from build123d import *

# Parameters (mm, degrees)
F1_DEPTH = 254


with BuildPart() as f1:
    # F0 (on Top) → F1 (new body)
    with BuildSketch(Plane.XY):
        with BuildLine():
            ThreePointArc((-29.842062, 64.568127), (-16.660152, 69.246382), (-2.831554, 71.348459))
            Line((-2.831554, 71.348459), (63.255093, 33.106133))
            ThreePointArc((63.255093, 33.106133), (68.338603, 20.057423), (70.860705, 6.282449))
            Line((70.860705, 6.282449), (70.630319, 6.282449))
            Line((70.630319, 6.282449), (62.698711, 6.291514))
            Line((62.698711, 6.291514), (62.698711, 3.370512))
            Line((62.698711, 3.370512), (70.62698, 3.361451))
            Line((70.62698, 3.361451), (71.05381, 3.361451))
            Line((71.05381, 3.361451), (71.05343, 2.472453))
            Line((71.05343, 2.472453), (71.051259, -2.607547))
            Line((71.051259, -2.607547), (72.340575, -2.607547))
            Line((72.340575, -2.607547), (72.340575, 2.472453))
            Line((72.340575, 2.472453), (73.630904, 2.472453))
            ThreePointArc((73.630904, 2.472453), (70.963492, 20.100215), (64.273057, 36.625686))
            Line((64.273057, 36.625686), (-0.291446, 73.98688))
            ThreePointArc((-0.291446, 73.98688), (-20.379161, 70.861714), (-38.925678, 62.53647))
            Line((-38.925678, 62.53647), (-38.293981, 61.433763))
            Line((-38.293981, 61.433763), (-33.886026, 63.958903))
            Line((-33.886026, 63.958903), (-33.259961, 62.866025))
            ThreePointArc((-33.259961, 62.866025), (-32.867158, 63.073001), (-32.473114, 63.277605))
            Line((-32.473114, 63.277605), (-32.256725, 62.907915))
            Line((-32.256725, 62.907915), (-28.302588, 56.041036))
            Line((-28.302588, 56.041036), (-25.77126, 57.498644))
            Line((-25.77126, 57.498644), (-29.725397, 64.365523))
            Line((-29.725397, 64.365523), (-29.842062, 64.568127))
        make_face()
    extrude(amount=F1_DEPTH)


solid = f1.part
Read the model definition and answer for the solid it produces. Units are mm, in the model's axes. A direction names the side the tool comes from. Give positions to 0.01 mm unless a question says otherwise; leave off trailing zeros. Loops run counter-clockwise (first coordinate to the right, second up) from the corner with the lowest first, then second, coordinate; pieces in that order, holes last. Notation, with made-up numbers: M -35,9.25 L -2,9.25 A23 cw -2,24.25 Z; hole C -17,-19.75 d9. An arc over 180 degrees is marked long. Write each question's results on one line, items separated by ' | '.
1. The mould has two halves that part along X. Classify faces 1 (the face through (-20.11, 70.94, 125.22)), 2 (the face through (72.341, 0, 125)), 3 (the face through (30, 53, 254)), 4 (the face through (-36.12, 62.68, 125.22)): pulls with the +X half, pulls with the -X half, needs draft (parallel to the pull), parting line crosses it, or undercut.
Values:
face 1: pulls with the -X half | face 2: pulls with the +X half | face 3: needs draft | face 4: undercut
2. Straight lines are drawn through the part: line 1 (X direction, y = 0.5, z = 45); line 2 (X direction, y = 65, z = 206); line 3 (X direction, y = 66, z = 89). For each, find the intervals that lie inside material, in ascending order. Write a range as [from, to].
Values:
line 1: x = [71.05, 72.34] | line 2: x = [-34.66, -28.9], [8.14, 15.24] | line 3: x = [-32.72, -26.56], [6.41, 13.51]
3. Given pin 1 (8 mm diameter, centred on y = 57.5, z = 74.5, fed in from -X); pin 2 (6 mm diameter, centred on x = -0.5, y = 64.5, fed in from -Z); pin 3 (1 mm diameter, centred on y = 66, z = 207, fed in from +X); pin 4 (5.5 mm diameter, centred on y = -1, z = 184, fed in from -X), each flat-ended and moving along its own axis, determine where each tip first touches the part or whether it passes through.
Values:
pin 1: stops at x = -38.33 | pin 2: passes through | pin 3: stops at x = 14.37 | pin 4: stops at x = 71.05
4. Section A-A on z = 42.5 is taken. Give the vertices of the cut face in (x, y), plus the area to 3 significant figures.
Values:
outline: M -38.93,62.54 L -38.29,61.43 L -33.89,63.96 L -33.26,62.87 A73.64 cw -32.47,63.28 L -32.26,62.91 L -28.3,56.04 L -25.77,57.5 L -29.73,64.37 L -29.84,64.57 A73.66 cw -2.83,71.35 L 63.26,33.11 A73.66 cw 70.86,6.28 L 70.63,6.28 L 62.7,6.29 L 62.7,3.37 L 70.63,3.36 L 71.05,3.36 L 71.05,-2.61 L 72.34,-2.61 L 72.34,2.47 L 73.63,2.47 A76.2 ccw 64.27,36.63 L -0.29,73.99 A76.2 ccw Z | area: 502 mm^2
5. Section C-C on x = 20 is taken. Give the vertices of the cut face in (y, z), plus the area to 3 significant figures.
Values:
outline: M 58.14,0 L 62.24,0 L 62.24,254 L 58.14,254 Z | area: 1,040 mm^2
6. Section B-B on y = 41 is taken. Give the vertices of the cut face in (x, z), plus the area to 3 significant figures.
Values:
outline: M 49.61,0 L 56.71,0 L 56.71,254 L 49.61,254 Z | area: 1,800 mm^2
7. A tool of negligible diameter and unlimited length cuts with its end or side. For faces 5 (the face through (-30.307, 59.523, 125.222)), 6 (the face through (32.443, 55.045, 125.222)), from which of +Z, -Z, +X, -X, +Y, -Y can it reach the whole face along a straight path? Write none if from no direction.
Values:
face 5: +Z, -Z, -Y | face 6: +Z, -Z, +X, +Y
